Design review of the part built by this model. Coordinates are the model's own, in mm. Face numbers are marked on the shaded views. A direction names the side the tool comes from. Give positions to 0.01 mm unless a question says otherwise; leave off trailing zeros. Order: outer loops, then holes, each group sorted by start corner. A loop starts at its lowest first (then second) coordinate and runs counter-clockwise, first axis right, second up. Notation, with made-up numbers: (10.25, 47.25) -> (39.25, 47.25) arc R18 cw to (39.25, 73.25) -> close; hole circle Ø6 at (-39.5, 9.5). An arc over 180 degrees is marked (long way). Answer in a Markdown table with one row per item. Add a question column.
```python
from build123d import *

# Parameters (mm, degrees)
SKETCH_1_W          = 6
SKETCH_1_H          = 2
EXTRUDE_1_DEPTH     = 2
SKETCH_2_W          = 2
SKETCH_2_H          = 2
EXTRUDE_2_DEPTH     = 4
CUT_EXTRUDE_1_DEPTH = 4


with BuildPart() as part:
    # 草图1 → 凸台-拉伸1 (new body)
    with BuildSketch(Plane.XY):
        Rectangle(SKETCH_1_W, SKETCH_1_H)
    extrude(amount=EXTRUDE_1_DEPTH)

    # 草图2 → 凸台-拉伸2 (add)
    with BuildSketch(Plane(origin=(0, 0, 0), x_dir=(-1, 0, 0), z_dir=(0, 0, -1))):
        Rectangle(SKETCH_2_W, SKETCH_2_H)
    extrude(amount=EXTRUDE_2_DEPTH)

    # 草图3 → 切除-拉伸1 (cut)
    with BuildSketch(Plane(origin=(0, 1, 0), x_dir=(1, 0, 0), z_dir=(0, 1, 0))):
        Polygon((-1, 3.79771899), (-0.830611616, 4), (-0.589050738, 3.79771899), (-0.387722732, 4), (-0.184484207, 3.79771899), (0, 4), (0.221794632, 3.79771899), (0.406278839, 4), (0.628073471, 3.79771899), (0.812557678, 4), (1, 3.829048964), (1.133730845, 3.829048964), (1.133730845, 4.163918303), (-1.101555404, 4.163918303), (-1.101555404, 3.79771899), align=None)
    extrude(amount=-CUT_EXTRUDE_1_DEPTH, mode=Mode.SUBTRACT)


solid = part.part
```
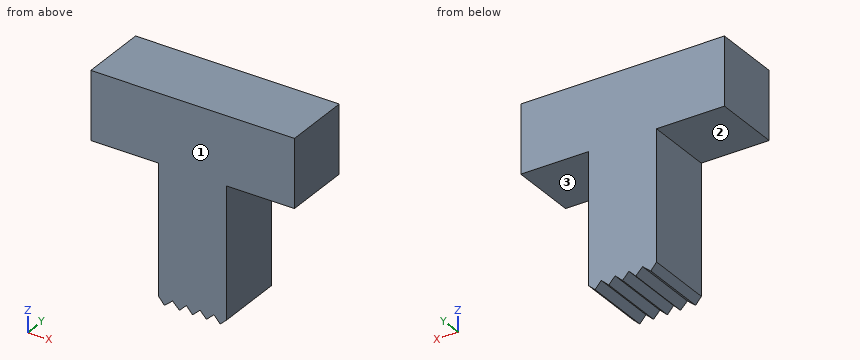
1) Add section C-C, the plane x = -1.2. Write out the cut boundary in (y, z).
2) Add section A-A, the plane y = -0.35. Write out the cut boundary in (x, z).
3) For L1, parallel to X at y = 0.45, z = -0.5; L2, parallel to Z at x = -2.1, y = 0.05; L3, parallel to Z at x = 0.05, y = 0.45, list the stretches that pass through material, from the lowest coordinate up.
4) Machinability: for the marked faces 1, 2 and 3, which of the approach directions +Z, -Z, +X, -X, +Y, -Y give a long, thin tool a straight path to every point of the face, cutting with its end or side? Answer none if there is none.
5) Clearance check with flat-ended pins moving along their axes: P1, Ø1, axis at y = 0, z = -2.5, coming from the -X side; P2, Ø1, axis at y = -0.5, z = -2, coming from the +X side. State where each tip first meets the part, or that it passes through.
6) Add section B-B, the plane z = -0.8. Write out the cut boundary in (x, y), and give its area (3 significant figures).
Verdict:
| question | item | result |
|---|---|---|
| 1 | outline | (-1, 0) -> (1, 0) -> (1, 2) -> (-1, 2) -> close |
| 2 | outline | (-3, 0) -> (-1, 0) -> (-1, -3.8) -> (-0.83, -4) -> (-0.59, -3.8) -> (-0.39, -4) -> (-0.18, -3.8) -> (0, -4) -> (0.22, -3.8) -> (0.41, -4) -> (0.63, -3.8) -> (0.81, -4) -> (1, -3.83) -> (1, 0) -> (3, 0) -> (3, 2) -> (-3, 2) -> close |
| 3 | L1 | x = -1 to 1 |
| 3 | L2 | z = 0 to 2 |
| 3 | L3 | z = -3.95 to 2 |
| 4 | face 1 | +Z, -Z, +X, -X, -Y |
| 4 | face 2 | -Z, -X, +Y, -Y |
| 4 | face 3 | -Z, +X, +Y, -Y |
| 5 | P1 | stops at x = -1 |
| 5 | P2 | stops at x = 1 |
| 6 | outline | (-1, -1) -> (1, -1) -> (1, 1) -> (-1, 1) -> close |
| 6 | area | 4.00 mm2 |
